Part model, mm, in its own coordinate system. Face numbers are marked on the shaded views. Round coordinates to 2 decimals unless told otherwise and drop trailing zeros. Loops run counter-clockwise (first coordinate to the right, second up) from the corner with the lowest first, then second, coordinate; pieces in that order, holes last. Notation, with made-up numbers: M 67,-11 L 91,-11 A6 cw 91,-6 Z; hole C -39,65.25 d10. An arc over 180 degrees is marked long. Write each question's results on one line, items separated by ' | '.
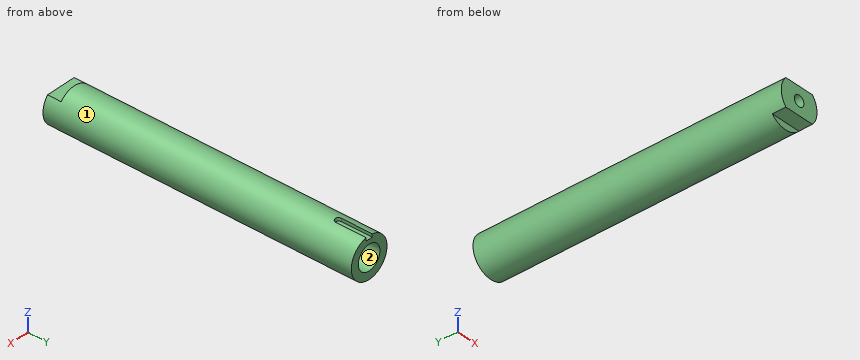
from build123d import *

# Parameters (mm, degrees)
SKETCH1_R                       = 9.5
BOSS_EXTRUDE1_DEPTH             = 144.78
CUT_EXTRUDE1_DEPTH              = 6.35
TAP_DRILL_FOR_1_4_20_TAP1_D     = 5.1054
TAP_DRILL_FOR_1_4_20_TAP1_DEPTH = 31.75
TAP_DRILL_FOR_1_4_20_TAP1_TIP   = 1.533816902
TAP_DRILL_FOR_1_2_20_TAP1_D     = 11.50874
TAP_DRILL_FOR_1_2_20_TAP1_DEPTH = 31.75
TAP_DRILL_FOR_1_2_20_TAP1_TIP   = 3.45757432
CUT_EXTRUDE2_DEPTH              = 1.5875


with BuildPart() as part:
    # Sketch1 → Boss-Extrude1 (new body)
    with BuildSketch(Plane(origin=(0, 0, 0), x_dir=(1, 0, 0), z_dir=(0, 1, 0))):
        Circle(SKETCH1_R)
    extrude(amount=BOSS_EXTRUDE1_DEPTH)

    # Sketch2 → Cut-Extrude1 (cut)
    with BuildSketch(Plane(origin=(0, 0, 0), x_dir=(-1, 0, 0), z_dir=(0, -1, 0))):
        with BuildLine():
            Line((7.065939428, -6.35), (-7.065939428, -6.35))
            ThreePointArc((-7.065939428, -6.35), (0, -9.5), (7.065939428, -6.35))
        make_face()
        with BuildLine():
            Line((7.065939428, 6.35), (-7.065939428, 6.35))
            ThreePointArc((-7.065939428, 6.35), (0, 9.5), (7.065939428, 6.35))
        make_face()
    extrude(amount=-CUT_EXTRUDE1_DEPTH, mode=Mode.SUBTRACT)

    # Tap Drill for 1/4-20 Tap1
    with Locations(Plane(origin=(0, 0, 0), x_dir=(-1, 0, 0), z_dir=(0, -1, 0))):
        with Locations((0, 0)):
            Hole(TAP_DRILL_FOR_1_4_20_TAP1_D / 2, depth=TAP_DRILL_FOR_1_4_20_TAP1_DEPTH)
            with Locations((0, 0, -(TAP_DRILL_FOR_1_4_20_TAP1_DEPTH + TAP_DRILL_FOR_1_4_20_TAP1_TIP / 2))):  # 118° drill point
                Cone(0, TAP_DRILL_FOR_1_4_20_TAP1_D / 2, TAP_DRILL_FOR_1_4_20_TAP1_TIP, mode=Mode.SUBTRACT)

    # Tap Drill for 1/2-20 Tap1
    with Locations(Plane(origin=(0, 144.78, 0), x_dir=(1, 0, 0), z_dir=(0, 1, 0))):
        with Locations((0, 0)):
            Hole(TAP_DRILL_FOR_1_2_20_TAP1_D / 2, depth=TAP_DRILL_FOR_1_2_20_TAP1_DEPTH)
            with Locations((0, 0, -(TAP_DRILL_FOR_1_2_20_TAP1_DEPTH + TAP_DRILL_FOR_1_2_20_TAP1_TIP / 2))):  # 118° drill point
                Cone(0, TAP_DRILL_FOR_1_2_20_TAP1_D / 2, TAP_DRILL_FOR_1_2_20_TAP1_TIP, mode=Mode.SUBTRACT)

    # Sketch7 → Cut-Extrude2 (cut)
    with BuildSketch(Plane.XY.offset(9.5)):
        with BuildLine():
            Line((-1.5875, 130.4925), (-1.5875, 144.78))
            Line((-1.5875, 144.78), (1.5875, 144.78))
            Line((1.5875, 144.78), (1.5875, 130.4925))
            ThreePointArc((1.5875, 130.4925), (0, 128.905), (-1.5875, 130.4925))
        make_face()
    extrude(amount=-CUT_EXTRUDE2_DEPTH, mode=Mode.SUBTRACT)


solid = part.part
Item 1: Drop flat-ended pins along their axis: P1, Ø1.6, axis at y = 134, z = 8.5, coming from the +X side; P2, Ø4, axis at x = 0, z = 0, coming from the -Y side; P3, Ø3, axis at x = 3, z = -2, coming from the +Y side; P4, Ø3, axis at x = -7, z = -1, coming from the -Y side. Give the stop position or say it passes through.
Filled sheet:
P1: x = 5.56 | P2: y = 32.08 | P3: y = 112.64 | P4: y = 0
Item 2: Two-plate mould, pull along Z, no slides. Class the marked faces 1 and 2: +Z half, -Z half, draft (parallel to the pull), parting line (faces both ways), or undercut.
Filled sheet:
face 1: parting line | face 2: undercut
Item 3: Band-saw the part on B-B on y = 115. Give the cut face in (x, z), and give its area (3 significant figures).
Filled sheet:
outline: C 0,0 d19; hole C 0,0 d11.51 | area: 180 mm^2
Item 4: Band-saw the part on A-A on y = 39. Give the cut face in (x, z), and give its area (3 significant figures).
Filled sheet:
outline: C 0,0 d19 | area: 284 mm^2
Item 5: Wall check: L1, parallel to Z at x = 0, y = 13; L2, parallel to Z at x = 0, y = 122.5; L3, parallel to Y at x = 5.5, z = 7.25. Give the ranges that are in metal, low to high.
Filled sheet:
L1: -9.5 to -2.55, 2.55 to 9.5 | L2: -9.5 to -5.75, 5.75 to 9.5 | L3: 6.35 to 144.78
